Source: CAD feature listing. Evaluate the final solid. Frame: model axes, mm. Coordinates: 2 decimals unless noted, no trailing zeros. Loops run counter-clockwise (first coordinate to the right, second up) from the corner with the lowest first, then second, coordinate; pieces in that order, holes last.
```python
from build123d import *

# Parameters (mm, degrees)
SKETCH1_R           = 290
SKETCH1_R_2         = 157.5
BOSS_EXTRUDE1_DEPTH = 4
SKETCH2_R           = 6
CUT_EXTRUDE1_DEPTH  = 4
CIRPATTERN1_COUNT   = 8
SKETCH3_R           = 6
CUT_EXTRUDE2_DEPTH  = 4
CIRPATTERN2_COUNT   = 12


with BuildPart() as part:
    # Sketch1 → Boss-Extrude1 (new body)
    with BuildSketch(Plane(origin=(0, 0, 0), x_dir=(1, 0, 0), z_dir=(0, 1, 0))):
        with Locations(Location((0, 0, 0), (0, 0, 270))):
            Circle(SKETCH1_R)
        with Locations(Location((0, 0, 0), (0, 0, 270))):
            Circle(SKETCH1_R_2, mode=Mode.SUBTRACT)
    extrude(amount=BOSS_EXTRUDE1_DEPTH)

    # Sketch2 → Cut-Extrude1 (cut)
    with BuildSketch(Plane(origin=(0, 4, 0), x_dir=(1, 0, 0), z_dir=(0, 1, 0))):
        with Locations(Location((182.5, 0, 0), (0, 0, 270))):
            Circle(SKETCH2_R)
    cut_extrude1 = extrude(amount=-CUT_EXTRUDE1_DEPTH, mode=Mode.SUBTRACT)

    # CirPattern1: Cut-Extrude1 ×8 about axis
    cirpattern1_axis = Axis((0, 0, 0), (0, 1, 0))
    for i in range(1, CIRPATTERN1_COUNT):
        add(cut_extrude1.rotate(cirpattern1_axis, i * 360 / CIRPATTERN1_COUNT), mode=Mode.SUBTRACT)

    # Sketch3 → Cut-Extrude2 (cut)
    with BuildSketch(Plane(origin=(0, 4, 0), x_dir=(1, 0, 0), z_dir=(0, 1, 0))):
        with Locations(Location((275, 0, 0), (0, 0, 270))):
            Circle(SKETCH3_R)
    cut_extrude2 = extrude(amount=-CUT_EXTRUDE2_DEPTH, mode=Mode.SUBTRACT)

    # CirPattern2: Cut-Extrude2 ×12 about axis
    cirpattern2_axis = Axis((0, 0, 0), (0, 1, 0))
    for i in range(1, CIRPATTERN2_COUNT):
        add(cut_extrude2.rotate(cirpattern2_axis, i * 360 / CIRPATTERN2_COUNT), mode=Mode.SUBTRACT)


solid = part.part
```
Q1. Section query A-A on z = 29. Return the cut outline in (x, y), then the cut area to 3 significant figures.
Q2. First-contact query: pin 1 Ø9.5 at (x, z) = (137.5, -238.16) entering from +Y; pin 2 Ø19 at (x, z) = (129.05, -129.05) entering from -Y. Flat tips, straight axial feed; report the tip coordinate or a pass-through.
Q3. Draft query along Z for faces 1 (the flat face through (-189, 4, -4)), 2 (the cylindrical face through (-153.755, 1.972, -34.143)), 3 (the cylindrical face through (87.108, 1.972, 276.608)). Return one class per face: released by +Z, released by -Z, zero draft, split by the parting line, or undercut.
Q4. Section query D-D on z = 214. Return the cut outline in (x, y), then the cut area to 3 significant figures.
Q5. Material intervals for line 1 along X through (y, z) = (1.6, -137.5); line 2 along X through (y, z) = (2.1, -126); line 3 along Z through (x, y) = (141.5, 2.35), sorted ascending.
Q6. Section query B-B on y = 0.8. Count the separate pieces of the cut face and the enclosed holes in it, then the cut area to 3 significant figures.
Q7. Section query C-C on x = -66. Return the cut outline in (y, z).
Resolved:
1. outline: (-288.55, 0) - (-154.81, 0) - (-154.81, 4) - (-288.55, 4) - close; (154.81, 0) - (288.55, 0) - (288.55, 4) - (154.81, 4) - close
1. area: 1,070 mm2
2. pin 1: passes through
2. pin 2: stops at y = 0
3. face 1: zero draft
3. face 2: undercut
3. face 3: split by the parting line
4. outline: (-195.71, 0) - (195.71, 0) - (195.71, 4) - (-195.71, 4) - close
4. area: 1,570 mm2
5. line 1: x = -255.33 to -244.16, -232.16 to -76.81, 76.81 to 232.16, 244.16 to 255.33
5. line 2: x = -261.2 to -134.22, -123.88 to -94.5, 94.5 to 123.88, 134.22 to 261.2
5. line 3: z = -253.14 to -242.63, -233.68 to -69.17, 69.17 to 233.68, 242.63 to 253.14
6. separate pieces: 1
6. enclosed holes: 21
6. area: 184,000 mm2
7. outline: (0, -282.39) - (4, -282.39) - (4, -143) - (0, -143) - close; (0, 143) - (4, 143) - (4, 282.39) - (0, 282.39) - close
